Source: CAD feature listing. Evaluate the final solid. Frame: model axes, mm. A direction names the side the tool comes from. Coordinates: 2 decimals unless noted, no trailing zeros. Write each loop counter-clockwise with the first axis right and the second up, starting at its lowest first coordinate (ties: lowest second). Pieces come first, ordered by that corner, then holes. Notation, with made-up numbers: M 19.25,-7 L 47.25,-7 A20 cw 47.25,19 Z; hole C 2,46 d4. An arc over 180 degrees is marked long. Write item = value, one per line. Start each with the question number.
1. Pull-direction query (Z, two-part tool) for faces 5 (the face through (-1, 0, 19)), 6 (the face through (-1, -50, 0)), 7 (the face through (0, -99, 14.021)), 8 (the face through (0, -3, 33.02)); classes: pulls with the +Z half, pulls with the -Z half, needs draft (parallel to the pull), parting line crosses it, or undercut.
2. Section query C-C (x = 24.5). Output: boundary loops of the cut face in (y, z).
3. Access query for faces 1 (the face through (0, -50, 7.62)), 2 (the face through (-33.02, -50, 36)), 3 (the face through (-38.1, -50, 19)), 4 (the face through (0, -99, 21.997)). Directions: +Z, -Z, +X, -X, +Y, -Y. A direction counts if a zero-diameter tool reaches every point of the face in a straight line with its end or side. Return the directions, or none.
4. Section query D-D (z = 16.5). Output: boundary loops of the cut face in (x, y).
5. Line query: line 1 along Y through (x, z) = (12.5, 23); line 2 along X through (y, z) = (-71.5, 15.5); line 3 along Z through (x, y) = (-18, -62.5). Output: solid intervals per line, ascending.
6. Pin query (flat end, axial travel): pin 1 Ø5.5 at (x, y) = (13.5, -3) entering from +Z. Return the tip coordinate at first contact, or that it passes through.
7. Section query A-A (x = -5). Output: boundary loops of the cut face in (y, z).
```python
from build123d import *

# Parameters (mm, degrees)
F0_W     = 66.04
F0_H     = 27.94
F1_DEPTH = 101.6
F2_W     = 66.040002
F2_H     = 91.44
F3_DEPTH = 25.4
F4_W     = 19.812
F4_H     = 7.9756
F5_DEPTH = 12.7


with BuildPart() as f1:
    # F0 (on Front) → F1 (new body)
    with BuildSketch(Plane.XZ):
        Polygon((-38.1, 0), (-33.02, 0), (-33.02, 5.08), (-33.02, 33.02), (-33.02, 38.1), (-38.1, 38.1), align=None)
        Polygon((-33.02, 0), (0, 0), (33.02, 0), (33.02, 5.08), (-33.02, 5.08), align=None)
        Polygon((33.02, 5.08), (33.02, 0), (38.1, 0), (38.1, 38.1), (33.02, 38.1), (33.02, 33.02), align=None)
        with Locations((0, 19.05)):
            Rectangle(F0_W, F0_H)
    extrude(amount=F1_DEPTH)

    # F2 (on face) → F3 (cut)
    with BuildSketch(Plane.XY.offset(33.02)):
        with Locations((0, -50.8)):
            Rectangle(F2_W, F2_H)
    extrude(amount=-F3_DEPTH, mode=Mode.SUBTRACT)

    # F4 (on face) → F5 (cut)
    with BuildSketch(Plane.XZ.offset(101.6)):
        with Locations((0, 18.008964)):
            Rectangle(F4_W, F4_H)
    extrude(amount=-F5_DEPTH, mode=Mode.SUBTRACT)


solid = f1.part
```
Results are:
q1.face_5 = needs draft
q1.face_6 = pulls with the -Z half
q1.face_7 = undercut
q1.face_8 = pulls with the +Z half
q2.outline = M -101.6,0 L 0,0 L 0,33.02 L -5.08,33.02 L -5.08,7.62 L -96.52,7.62 L -96.52,33.02 L -101.6,33.02 Z
q3.face_1 = +Z
q3.face_2 = +Z, +Y, -Y
q3.face_3 = +Z, -Z, -X, +Y, -Y
q3.face_4 = -Y
q4.outline = M -38.1,-101.6 L -9.91,-101.6 L -9.91,-96.52 L -33.02,-96.52 L -33.02,-5.08 L 33.02,-5.08 L 33.02,-96.52 L 9.91,-96.52 L 9.91,-101.6 L 38.1,-101.6 L 38.1,0 L -38.1,0 Z
q5.line_1 = -101.6 to -96.52, -5.08 to 0
q5.line_2 = -38.1 to -33.02, 33.02 to 38.1
q5.line_3 = 0 to 7.62
q6.pin_1 = 33.02
q7.outline = M -101.6,0 L 0,0 L 0,33.02 L -5.08,33.02 L -5.08,7.62 L -96.52,7.62 L -96.52,14.02 L -101.6,14.02 Z; M -101.6,22 L -96.52,22 L -96.52,33.02 L -101.6,33.02 Z
